Autodesk Inventor part; units mm, degrees
ref_plane "YZ Plane" through (0, 0, 0) normal (1, 0, 0) x (0, 1, 0)
ref_plane "XZ Plane" through (0, 0, 0) normal (0, 1, 0) x (-1, 0, 0)
ref_plane "XY Plane" through (0, 0, 0) normal (0, 0, 1) x (1, 0, 0)
sketch "Sketch1" plane through (0, 0, 0) normal (1, 0, 0) x (0, 1, 0)
  line L0 (0, 0) -> (38.75, 0)
  line L1 (38.75, 0) -> (38.75, -38.75)
  line L2 (38.75, -38.75) -> (0, -38.75)
  line L3 (0, -38.75) -> (0, 0)
  line L4 (0, -19.375) -> (19.375, -19.375)
  circle A0 centre (19.375, -19.375) radius 16
  dimension "d0" = 38.75
  dimension "d1" = 38.75
  dimension "d2" = 32
extrude "Extrusion1" add sketch "Sketch1" along normal blind 1
properties part number "Mag_Shield_front"
Geometry: final body of the model. Coordinates: model frame, mm. Coordinates: 2 decimals unless noted, no trailing zeros. Order: outer loops, then holes, each group sorted by start corner. A loop starts at its lowest first (then second) coordinate and runs counter-clockwise, first axis right, second up. Notation, with made-up numbers: M 59,50.5 L 66,50.5 A30 cw 66,77.5 Z; hole C 60,60.5 d6. An arc over 180 degrees is marked long. One line per question, with ' | ' between items. Start each with the question number.
Item 1: Cut plane B-B, the plane z = -20. Return the cut outline in (x, y).
Item 2: Draft query along Z for faces 1 (the flat face through (0.5, 38.75, -19.1)), 2 (the flat face through (0.5, 19.6, -38.75)), 3 (the flat face through (0.5, 19.1, 0)), 4 (the cylindrical face through (0.493, 15.907, -3.755)). Return one class per face: released by +Z, released by -Z, zero draft, split by the parting line, or undercut.
Item 3: Cut plane C-C, the plane x = 0.7. Return the cut outline in (y, z) (3 decimals), then the cut area to 3 significant figures.
Item 4: Pin query (flat end, axial travel): pin 1 Ø8 at (y, z) = (31, -28.5) entering from -X. Return the tip coordinate at first contact, or that it passes through.
Item 5: Ray query, probe 1 along Y at (x, z) = (0.1, -19.5); probe 2 along Z at (x, y) = (0.4, 6.5); probe 3 along Y at (x, z) = (0.9, -32). Return the intervals inside material, ascending. Write a range as [from, to].
Item 6: Cut plane A-A, the plane y = 13.5. Return the cut outline in (x, z).
A:
1) outline: M 0,0 L 1,0 L 1,3.39 L 0,3.39 Z; M 0,35.36 L 1,35.36 L 1,38.75 L 0,38.75 Z
2) face 1: zero draft | face 2: released by -Z | face 3: released by +Z | face 4: undercut
3) outline: M 0,-38.75 L 38.75,-38.75 L 38.75,0 L 0,0 Z; hole C 19.375,-19.375 d32 | area: 697 mm2
4) pin 1: stops at x = 0
5) probe 1: y = [0, 3.38], [35.37, 38.75] | probe 2: z = [-38.75, -28.87], [-9.88, 0] | probe 3: y = [0, 9.55], [29.2, 38.75]
6) outline: M 0,-38.75 L 1,-38.75 L 1,-34.26 L 0,-34.26 Z; M 0,-4.49 L 1,-4.49 L 1,0 L 0,0 Z
